CAD build for the part. Positions are in the model's coordinates, mm. Face numbers are marked on the shaded views. A direction names the side the tool comes from. Round coordinates to 2 decimals unless told otherwise and drop trailing zeros. Order: outer loops, then holes, each group sorted by start corner. A loop starts at its lowest first (then second) coordinate and runs counter-clockwise, first axis right, second up. Notation, with made-up numbers: M 51,30.25 L 56,30.25 A32 cw 56,63.25 Z; hole C 56.25,40 d9. An arc over 180 degrees is marked long. Answer as CSV lines item,"result". Start each with the question number.
Autodesk Inventor part; units mm, degrees
ref_plane "Plano de trabalho1" through (131, -3, -14) normal (0, 0, -1) x (-1, 0, 0)
ref_plane "YZ Plane" through (0, 0, 0) normal (1, 0, 0) x (0, 1, 0)
ref_plane "XZ Plane" through (0, 0, 0) normal (0, 1, 0) x (-1, 0, 0)
sketch "Esboço1" plane through (0, 0, 0) normal (0, 1, 0) x (-1, 0, 0)
  line L0 (-93, -3) -> (0, -3)
  line L1 (0, -25) -> (-58, -25)
  line L2 (-93, 0) -> (-93, -28)
  line L3 (-93, -28) -> (-83, -28)
  line L4 (-55, -28) -> (0, -28)
  line L5 (0, -28) -> (0, 0)
  line L6 (0, 0) -> (-93, 0)
  line L7 (-55, -28) -> (-55, -53)
  line L8 (-55, -53) -> (-93, -53)
  line L9 (-93, -53) -> (-93, -50)
  line L10 (-93, -50) -> (-58, -50)
  line L11 (-58, -50) -> (-58, -25)
  arc A0 (-83, -50) -> (-58, -25) centre (-83, -25) ccw
  arc A1 (-83, -28) -> (-80, -25) centre (-83, -25) ccw
  line L12 (-93, -25) -> (-80, -25)
  line L13 (0, 0) -> (3, 0)
  line L14 (3, 0) -> (3, -28)
  line L15 (3, -28) -> (0, -28)
  line L16 (-83, -28) -> (-83, -25)
  line L17 (-93, -50) -> (-93, -28)
  line L18 (0, -3) -> (3, -3)
  line L19 (0, -25) -> (3, -25)
  line L20 (-93, -3) -> (-186, -3)
  line L21 (-186, -25) -> (-128, -25)
  line L22 (-131, -28) -> (-186, -28)
  line L23 (-186, -28) -> (-186, 0)
  line L24 (-186, 0) -> (-93, 0)
  line L25 (-131, -28) -> (-131, -53)
  line L26 (-131, -53) -> (-93, -53)
  line L27 (-93, -50) -> (-128, -50)
  line L28 (-128, -50) -> (-128, -25)
  line L29 (-186, 0) -> (-189, 0)
  line L30 (-189, 0) -> (-189, -28)
  line L31 (-189, -28) -> (-186, -28)
  line L32 (-186, -3) -> (-189, -3)
  line L33 (-186, -25) -> (-189, -25)
  line L34 (-93, -28) -> (-128, -28)
  line L35 (-93, -25) -> (-128, -25)
  line L36 (-106, -50) -> (-106, -28)
  point P0 (-93, -14)
  point P1 (-93, -51.5)
  point P2 (-83, -28)
  dimension "d7" = 22
  dimension "d9" = 3
  dimension "d10" = 3
  dimension "d13" = 3
  dimension "d14" = 3
  dimension "d16" = 22
  dimension "d20" = 22
  dimension "d21" = 80
  dimension "d29" = 3
  dimension "d31" = 10
  dimension "d39" = 22
extrude "Extrusão1" add sketch "Esboço1" against normal blind 3 contours L20 L23 L24 L2 | L2 L35 L21 L23 L20 | L2 L34 L28 L35 | L32 L30 L29 L23 | L23 L33 L30 L32 | L17 L27 L36 L34 | L28 L27 L9 L26 L25 L22 L23 L21 | L23 L31 L30 L33
extrude "Extrusão2" add sketch "Esboço1" along normal blind 10 contours L20 L23 L24 L2 | L2 L34 L28 L35 | L32 L30 L29 L23 | L28 L27 L9 L26 L25 L22 L23 L21 | L23 L31 L30 L33
sketch "Esboço2" plane through (93, -3, 0) normal (0, 0, 1) x (1, 0, 0)
  line L0 (0, 13) -> (96, 13)
  line L1 (96, 0) -> (0, 0)
  line L2 (96, 0) -> (115.9239, 1.7431)
  line L3 (96, 0) -> (116, 0) construction
  line L4 (115.9239, 1.7431) -> (114.7952, 14.6444)
  line L5 (114.7952, 14.6444) -> (96, 13)
  line L6 (96, 0) -> (96, 13)
  line L7 (96, 0) -> (96, 13)
  dimension "d32" = 20
  dimension "d33" = 5
extrude "Extrusão4" add sketch "Esboço2" against normal up to surface (28 mm away)
ref_plane "Plano de trabalho1" through (131, -3, -14) normal (0, 0, -1) x (-1, 0, 0)
sketch "Esboço3" plane through (131, -3, -14) normal (0, 0, -1) x (-1, 0, 0)
  line L0 (-76.7952, 14.6444) -> (-58, 13)
  line L1 (38, 13) -> (-58, 13)
  line L2 (-77.6667, 4.6824) -> (-58.4366, 3)
  line L3 (-58.4366, 3) -> (38, 3)
  line L4 (-77.9239, 1.7431) -> (-76.7952, 14.6444)
  line L5 (-76.7952, 14.6444) -> (-77.6667, 4.6824)
  line L6 (-58, 3) -> (-58, 13)
  line L7 (-76.7952, 14.6444) -> (-58, 13)
  line L8 (-58, 13) -> (-58, 3)
  dimension "d40" = 10
extrude "Extrusão5" cut sketch "Esboço3" along normal mid plane 22
equation "\"d9\" = mdf"
equation "\"d10\" = mdf"
equation "\"d13\" = mdf"
equation "\"d14\" = mdf"
equation "\"mdf\" = 3"
equation "\"margem\" = 1"
properties part number "Trilho 5 min"
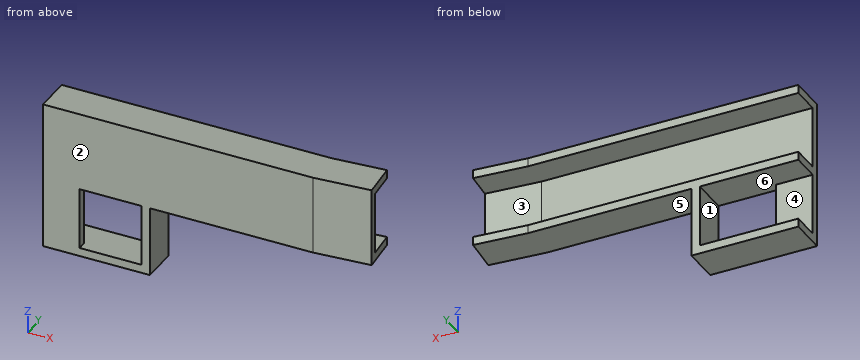
Q1. Band-saw the part on C-C, the plane y = 5.75. Write the cut outline in (x, z), then the cut area to 3 significant figures.
Q2. Band-saw the part on D-D, the plane z = -6.5. Write the cut outline in (x, y), then the cut area to 3 significant figures.
Q3. Band-saw the part on A-A, the plane x = 120. Write the cut outline in (y, z).
Q4. Probe line 1 along Z through (x, y) = (109.5, 0.25); line 2 along Z through (x, y) = (144, 3.25); line 3 along X through (y, z) = (2, -29.5). List the from-to ranges inside material, lowest first. Write a range as from..to.
Q5. Band-saw the part on B-B, the plane z = -31.5. Write the cut outline in (x, y), then the cut area to 3 significant figures.
Q6. Drop flat-ended pins along their axis: P1, Ø3, axis at y = 5.5, z = -30, coming from the +X side; P2, Ø3, axis at x = 162, y = 3, coming from the -Z side; P3, Ø6, axis at x = 132.5, z = -17, coming from the +Y side. Give the stop position or say it passes through.
Q7. Mould opens along X. For the marked faces 1, 2 and 3 say: +X half, -X half, draft (parallel to the pull), parting line (faces both ways), or undercut.
Q8. Tool access for the marked faces 4, 5 and 6: list every direction of +Z, -Z, +X, -X, +Y, -Y with a clear straight run to the whole face (end or side of a thin tool).
Answer:
1,outline,"M 93,-53 L 131,-53 L 131,-28 L 208.31,-28 L 208.31,-25 L 93,-25 L 93,-28 L 128,-28 L 128,-50 L 93,-50 Z; M 93,-3 L 208.31,-3 L 208.31,0 L 93,0 Z"
1,area,"872 mm^2"
2,outline,"M 93,-3 L 189,-3 L 208.92,-1.26 L 208.67,1.68 L 189.44,0 L 93,0 Z"
2,area,"347 mm^2"
3,outline,"M -3,-53 L 10,-53 L 10,-50 L -3,-50 Z; M -3,-28 L 10,-28 L 10,-25 L 0,-25 L 0,-3 L 10,-3 L 10,0 L -3,0 Z"
4,line 1,"z = -53..-50, -28..-25, -3..0"
4,line 2,"z = -28..-25, -3..0"
4,line 3,"x = 128..131"
5,outline,"M 93,-3 L 106,-3 L 106,0 L 93,0 Z; M 128,-3 L 131,-3 L 131,10 L 128,10 Z"
5,area,"78.0 mm^2"
6,P1,"stops at x = 131"
6,P2,"stops at z = -28"
6,P3,"stops at y = 0"
7,face 1,"undercut"
7,face 2,"draft"
7,face 3,"-X half"
8,face 4,"-X, +Y"
8,face 5,"-Z, +X, +Y, -Y"
8,face 6,"+Y"
